Part model, mm, in its own coordinate system. A direction names the side the tool comes from. Give positions to 0.01 mm unless a question says otherwise; leave off trailing zeros. Order: outer loops, then holes, each group sorted by start corner. A loop starts at its lowest first (then second) coordinate and runs counter-clockwise, first axis right, second up. Notation, with made-up numbers: (-4, -34.75) - (10, -34.75) arc R27 ccw to (10, 2.25) - close; hole circle Ø7 at (62, 33.25). An arc over 180 degrees is marked (long way). One line per item, written item: value.
```python
from build123d import *

# Parameters (mm, degrees)
F0_W     = 44.9535958469
F0_H     = 55.96075207
F1_DEPTH = 25.4
F2_R     = 5.08
F7_DEPTH = 2.6416
F8_R     = 2.286


# Not quite as in the source:
# - the program builds the solid bodies; features that only make, move or delete a surface that nothing else refers to are left out


with BuildPart() as f1:
    # F0 (on Front) → F1 (new body)
    with BuildSketch(Plane.XZ):
        with Locations((-22.4767979234, 27.980376035)):
            Rectangle(F0_W, F0_H)
    extrude(amount=F1_DEPTH)

    # F2
    f2_edges = [f1.edges().sort_by_distance(p)[0] for p in [
        (-44.953596, -25.4, 27.980376),
        (-44.953596, 0, 27.980376),
        (0, -25.4, 27.980376),
        (0, 0, 27.980376),
    ]]
    fillet(f2_edges, radius=F2_R)

    # F6 (on face) → F7 (join)
    with BuildSketch(Plane.XY.offset(55.96075207)):
        Polygon((-36.077086072, -5.0010341604), (-40.522086072, -12.7), (-36.077086072, -20.3989658396), (-27.187086072, -20.3989658396), (-22.742086072, -12.7), (-27.187086072, -5.0010341604), align=None)
        Polygon((-34.807086072, -18.199261314), (-37.982086072, -12.7), (-34.807086072, -7.200738686), (-28.457086072, -7.200738686), (-25.282086072, -12.7), (-28.457086072, -18.199261314), align=None, mode=Mode.SUBTRACT)
    extrude(amount=F7_DEPTH)

    # F8
    f8_edges = [f1.edges().sort_by_distance(p)[0] for p in [
        (-22.476798, -25.4, 55.960752),
    ]]
    fillet(f8_edges, radius=F8_R)


solid = f1.part
```
1) Cut at A-A, the plane z = 10. Give the cut face in (x, y), then the cut area to 3 significant figures.
Outcome:
outline: (-44.95, -20.32) arc R5.08 ccw to (-39.87, -25.4) - (-5.08, -25.4) arc R5.08 ccw to (0, -20.32) - (0, -5.08) arc R5.08 ccw to (-5.08, 0) - (-39.87, 0) arc R5.08 ccw to (-44.95, -5.08) - close
area: 1,120 mm^2
2) Cut at B-B, the plane x = -11.5. Give the cut face in (y, z), then the cut area to 3 significant figures.
Outcome:
outline: (-25.4, 0) - (0, 0) - (0, 53.67) arc R2.29 ccw to (-2.29, 55.96) - (-23.11, 55.96) arc R2.29 ccw to (-25.4, 53.67) - close
area: 1,420 mm^2
3) Cut at C-C, the plane y = -8.75. Give the cut face in (x, z), then the cut area to 3 significant figures.
Outcome:
outline: (-44.95, 0) - (0, 0) - (0, 53.67) arc R2.29 ccw to (-2.29, 55.96) - (-25.02, 55.96) - (-25.02, 58.6) - (-27.56, 58.6) - (-27.56, 55.96) - (-35.7, 55.96) - (-35.7, 58.6) - (-38.24, 58.6) - (-38.24, 55.96) - (-42.67, 55.96) arc R2.29 ccw to (-44.95, 53.67) - close
area: 2,530 mm^2
4) Which spindle directions (+Z, -Z, +X, -X, +Y, -Y) get a long thin tool onto all of the face, cutting with end or side? Do faces 1 (the flat face through (-32, -20.399, 57)), 2 (the flat face through (-24.933, -8.904, 57.263)), 3 (the flat face through (-26.9, -9.9, 57.3)), 4 (the flat face through (-32, -5.001, 57)). Say none if no direction does.
Outcome:
face 1: +Z, +X, -X, -Y
face 2: +Z, +X, +Y
face 3: +Z
face 4: +Z, +X, -X, +Y
5) Mould opens along X. For faces 5 (the flat face through (-36.37, -15.49, 57.26)), 6 (the cylindrical face through (-43.505, -1.528, 27.213)), 7 (the flat face through (-23, -13, 0)), 8 (the flat face through (-32, -13, 55.961)) say: released by +X, released by -X, zero draft, split by the parting line, or undercut.
Outcome:
face 5: undercut
face 6: released by -X
face 7: zero draft
face 8: undercut
6) Drill centre lines: line 1 along Z through (x, y) = (-11, -6.25); line 2 along Y through (x, z) = (-5, 47); line 3 along Y through (x, z) = (-1.5, 16). Where is each one in solid material? Low to high. Write a range as from..to.
Outcome:
line 1: z = 0..55.96
line 2: y = -25.4..0
line 3: y = -23.92..-1.48
7) Pin check, flat tips, straight feed: pin 1 (4 mm diameter, centred on x = -12, y = -4.5, fed in from +Z); pin 2 (6 mm diameter, centred on x = -37, y = -4.5, fed in from -Z); pin 3 (0.8 mm diameter, centred on x = -33, z = 58, fed in from -Y); pin 4 (3 mm diameter, centred on x = -33, z = 57, fed in from -Y). Stop position of each tip, or through.
Outcome:
pin 1: stops at z = 55.96
pin 2: stops at z = 0
pin 3: stops at y = -20.4
pin 4: stops at y = -24.49
